For this review, use the dimensioned drawing (mm, ordinates from the lowest corner) and the shaded views. A direction names the side the tool comes from. Give positions to 0.01 mm unless a question says otherwise; leave off trailing zeros. Write each loop counter-clockwise with the first axis right and the second up, starting at its lowest first coordinate (ties: lowest second). Pieces come first, ordered by that corner, then holes. Notation, with made-up numbers: M 43,18.25 L 54,18.25 A22 ccw 54,34.25 Z; hole C 75.25,-4.5 d8. An arc over 180 degrees is marked long. Answer in a Markdown table with one row per item.
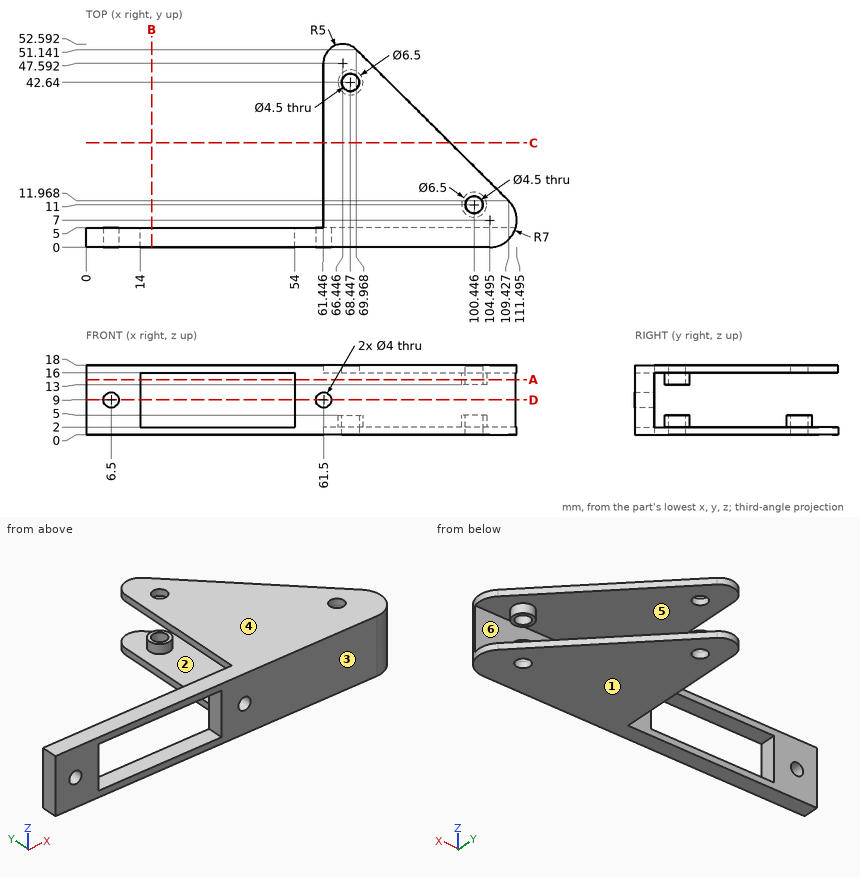
1) Add section D-D (z = 9). Write out the cut boundary in (x, y) (1 decimal).
Geometry says:
| item | result |
|---|---|
| outline | M 0,0 L 4.5,0 L 4.5,5 L 0,5 Z; M 8.5,0 L 14,0 L 14,5 L 8.5,5 Z; M 54,0 L 59.5,0 L 59.5,5 L 54,5 Z; M 63.5,0 L 104.5,0 A7 ccw 111.2,5 L 63.5,5 Z |
2) Add section C-C (y = 27). Write out the cut boundary in (x, z) (1 decimal).
Geometry says:
| item | result |
|---|---|
| outline | M 61.4,0 L 94.3,0 L 94.3,2 L 61.4,2 Z; M 61.4,16 L 94.3,16 L 94.3,18 L 61.4,18 Z |
3) Insertion check: P1, Ø24, axis at x = 82.5, y = 17.5, coming from the -Z side; P2, Ø1, axis at y = 20, z = 16.5, coming from the -X side; P3, Ø5, axis at y = 10, z = 6, coming from the +X side; P4, Ø5, axis at y = 40.5, z = 4, coming from the +X side. Each pin has a flat end and moves straight along its axis. Give the tip position at first contact, or say it passes through.
Geometry says:
| item | result |
|---|---|
| P1 | z = 0 |
| P2 | x = 61.45 |
| P3 | x = 103.7 |
| P4 | x = 82.2 |
4) To check wall thickness, follow probe 1 along Z at (x, y) = (63.5, 44); probe 2 along X at (y, z) = (11, 15.2) (1 decimal); probe 3 along X at (y, z) = (2.35, 9). State the ranges of each line that lie inside material, in increasing order. Write a range as [from, to].
Geometry says:
| item | result |
|---|---|
| probe 1 | [0, 2], [16, 18] |
| probe 2 | [97.2, 98.2], [102.7, 103.7] |
| probe 3 | [0, 4.5], [8.5, 14], [54, 59.5], [63.5, 109.73] |
5) Add section B-B (x = 17). Write out the cut boundary in (y, z), and give its area (3 significant figures).
Geometry says:
| item | result |
|---|---|
| outline | M 0,0 L 5,0 L 5,2 L 0,2 Z; M 0,16 L 5,16 L 5,18 L 0,18 Z |
| area | 20.0 mm^2 |
6) Add section A-A (z = 14.25). Count the separate pieces of the cut face and the enclosed holes in it.
Geometry says:
| item | result |
|---|---|
| separate pieces | 3 |
| enclosed holes | 1 |
7) The part is to be moulded in two halves that separate along Z. For the marked faces 3, 4, 5 and 6, say which applies: released by +Z, released by -Z, zero draft, split by the parting line, or undercut.
Geometry says:
| item | result |
|---|---|
| face 3 | zero draft |
| face 4 | released by +Z |
| face 5 | undercut |
| face 6 | undercut |
8) For the marked faces 1 and 2, list the 3-axis set-ups (+Z, -Z, +X, -X, +Y, -Y) from which the entire face can be reached by the end or side of a thin tool; tool diameter is ignored.
Geometry says:
| item | result |
|---|---|
| face 1 | -Z, +X, -X, +Y, -Y |
| face 2 | none |
